Verification items for the finished model (mm, model axes). Coordinates: 2 decimals unless noted, no trailing zeros. Order: outer loops, then holes, each group sorted by start corner. A loop starts at its lowest first (then second) coordinate and runs counter-clockwise, first axis right, second up. Notation, with made-up numbers: M 43,-16.5 L 99,-16.5 A26 ccw 99,20.5 Z; hole C -27,-2 d7. An arc over 180 degrees is marked long. Answer as a JSON object with one key per item and string values. Group by question number.
(1) Cross-section at A-A (x = 42.25). Enter the section's corners in (y, z).
(2) Gauge pin test, flat end, axial feed: pin 1 Ø3 at (x, z) = (42.25, -6) entering from +Y. Record the tip position at first contact, or that the pin passes through.
(3) Cross-section at D-D (x = 31.5). Enter the section's corners in (y, z).
(4) Cross-section at B-B (z = -6). Enter the section's corners in (x, y) (3 decimals).
(5) Material ranges on line 1 (Z direction, x = 20, y = 2.05) (3 decimals); line 2 (Z direction, x = 86.1, y = 2.35); line 3 (X direction, y = 2.7, z = -8.5), recorded low to high.
(6) Cross-section at C-C (y = 0.55). Count the separate pieces of the cut face and the enclosed holes in it, plus the area to 3 significant figures.
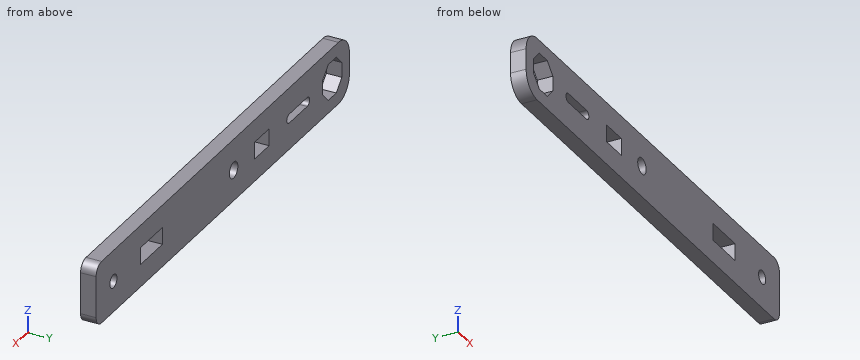
from build123d import *

# Parameters (mm, degrees)
SKETCH2_W           = 92.4
SKETCH2_H           = 12
BOSS_EXTRUDE1_DEPTH = 3
FILLET1_R           = 4
FILLET2_R           = 2
SKETCH3_R           = 1.55
SKETCH3_R_2         = 1.3
SKETCH3_W           = 5.4
SKETCH3_H           = 3
SKETCH3_W_2         = 8
CUT_EXTRUDE1_DEPTH  = 4
SKETCH4_W           = 5.4
SKETCH4_H           = 0.15
SKETCH4_W_2         = 8
CUT_EXTRUDE2_DEPTH  = 4


with BuildPart() as part:
    # Sketch2 → Boss-Extrude1 (new body)
    with BuildSketch(Plane(origin=(0, 0, 0), x_dir=(1, 0, 0), z_dir=(0, 1, 0))):
        with Locations((46.2, 6)):
            Rectangle(SKETCH2_W, SKETCH2_H)
    extrude(amount=BOSS_EXTRUDE1_DEPTH)

    # Fillet1
    fillet1_edges = [part.edges().sort_by_distance(p)[0] for p in [
        (0, 1.5, -12),
        (0, 1.5, 0),
    ]]
    fillet(fillet1_edges, radius=FILLET1_R)

    # Fillet2
    fillet2_edges = [part.edges().sort_by_distance(p)[0] for p in [
        (92.4, 1.5, -12),
        (92.4, 1.5, 0),
    ]]
    fillet(fillet2_edges, radius=FILLET2_R)

    # Sketch3 → Cut-Extrude1 (cut, through all)
    with BuildSketch(Plane(origin=(0, 3, 0), x_dir=(1, 0, 0), z_dir=(0, 1, 0))):
        with Locations((42.25, 6)):
            Circle(SKETCH3_R)
        with Locations((86.1, 6)):
            Circle(SKETCH3_R_2)
        Polygon((9.75, 7.449747468), (7.699747468, 9.5), (4.800252532, 9.5), (2.75, 7.449747468), (2.75, 4.550252532), (4.800252532, 2.5), (7.699747468, 2.5), (9.75, 4.550252532), align=None)
        with BuildLine():
            Line((15.4, 6.875), (22, 6.875))
            ThreePointArc((22, 6.875), (22.875, 6), (22, 5.125))
            Line((22, 5.125), (15.4, 5.125))
            ThreePointArc((15.4, 5.125), (14.525, 6), (15.4, 6.875))
        make_face()
        with Locations((32, 6)):
            Rectangle(SKETCH3_W, SKETCH3_H)
        with Locations((72.2, 6)):
            Rectangle(SKETCH3_W_2, SKETCH3_H)
    extrude(amount=-CUT_EXTRUDE1_DEPTH, mode=Mode.SUBTRACT)

    # Sketch4 → Cut-Extrude2 (cut, through all)
    with BuildSketch(Plane(origin=(0, 3, 0), x_dir=(1, 0, 0), z_dir=(0, 1, 0))):
        with Locations((32, 7.575)):
            Rectangle(SKETCH4_W, SKETCH4_H)
        with Locations((32, 4.425)):
            Rectangle(SKETCH4_W, SKETCH4_H)
        with Locations((72.2, 7.575)):
            Rectangle(SKETCH4_W_2, SKETCH4_H)
        with Locations((72.2, 4.425)):
            Rectangle(SKETCH4_W_2, SKETCH4_H)
    extrude(amount=-CUT_EXTRUDE2_DEPTH, mode=Mode.SUBTRACT)


solid = part.part
Taken from the geometry:
{
 "1": {"outline": "M 0,-12 L 3,-12 L 3,-7.55 L 0,-7.55 Z; M 0,-4.45 L 3,-4.45 L 3,0 L 0,0 Z"},
 "2": {"pin 1": "passes through"},
 "3": {"outline": "M 0,-12 L 3,-12 L 3,-7.65 L 0,-7.65 Z; M 0,-4.35 L 3,-4.35 L 3,0 L 0,0 Z"},
 "4": {"outline": "M 0,0 L 2.75,0 L 2.75,3 L 0,3 Z; M 9.75,0 L 14.525,0 L 14.525,3 L 9.75,3 Z; M 22.875,0 L 29.3,0 L 29.3,3 L 22.875,3 Z; M 34.7,0 L 40.7,0 L 40.7,3 L 34.7,3 Z; M 43.8,0 L 68.2,0 L 68.2,3 L 43.8,3 Z; M 76.2,0 L 84.8,0 L 84.8,3 L 76.2,3 Z; M 87.4,0 L 92.4,0 L 92.4,3 L 87.4,3 Z"},
 "5": {"line 1": "z = -12 to -6.875, -5.125 to 0", "line 2": "z = -12 to -7.3, -4.7 to 0", "line 3": "x = 0.03 to 3.8, 8.7 to 92.4"},
 "6": {"separate pieces": "1", "enclosed holes": "6", "area": "989 mm²"}
}
